Could you check a few things on this model? Use its own coordinates, in mm. A direction names the side the tool comes from. Coordinates: 2 decimals unless noted, no trailing zeros. Order: outer loops, then holes, each group sorted by start corner. A loop starts at its lowest first (then second) coordinate and runs counter-clockwise, first axis right, second up.
```python
from build123d import *

# Parameters (mm, degrees)
SKETCH1_W                     = 52
SKETCH1_H                     = 24
SKETCH1_R                     = 8.25
BOSS_EXTRUDE1_DEPTH           = 12
SKETCH2_R                     = 1
CUT_EXTRUDE1_DEPTH            = 32.048349393
SKETCH3_R                     = 1.75
CUT_EXTRUDE2_DEPTH            = 1
CUT_EXTRUDE3_DEPTH            = 5
FILLET3_R                     = 0.5
CHAMFER1_SIZE                 = 2.5
SKETCH5_W                     = 14
SKETCH5_H                     = 8
CUT_EXTRUDE4_DEPTH            = 5
FILLET4_R                     = 0.5
SKETCH6_W                     = 6.3
SKETCH6_H                     = 6.3
BOSS_EXTRUDE2_DEPTH           = 12
CSK_FOR_M3_SFHCS1_D           = 3
CSK_FOR_M3_SFHCS1_CSINK_D     = 6.3
CSK_FOR_M3_SFHCS1_CSINK_ANGLE = 90
CSK_FOR_M3_SFHCS2_D           = 3
CSK_FOR_M3_SFHCS2_DEPTH       = 109.998865618
CSK_FOR_M3_SFHCS2_CSINK_D     = 6.3
CSK_FOR_M3_SFHCS2_CSINK_ANGLE = 90


with BuildPart() as part:
    # Sketch1 → Boss-Extrude1 (new body)
    with BuildSketch(Plane(origin=(0, 0, 0), x_dir=(1, 0, 0), z_dir=(0, 1, 0))):
        Rectangle(SKETCH1_W, SKETCH1_H)
        with Locations(Location((12.75, 0, 0), (0, 0, 270))):
            Circle(SKETCH1_R, mode=Mode.SUBTRACT)
        with Locations(Location((-12.75, 0, 0), (0, 0, 270))):
            Circle(SKETCH1_R, mode=Mode.SUBTRACT)
    extrude(amount=BOSS_EXTRUDE1_DEPTH)

    # Sketch2 → Cut-Extrude1 (cut, through all)
    with BuildSketch(Plane(origin=(0, 12, 0), x_dir=(1, 0, 0), z_dir=(0, 1, 0))):
        with Locations(Location((-21.35, 8.85, 0), (0, 0, 270))):
            Circle(SKETCH2_R)
        with Locations(Location((21.35, 8.85, 0), (0, 0, 270))):
            Circle(SKETCH2_R)
        with Locations(Location((21.35, -8.85, 0), (0, 0, 270))):
            Circle(SKETCH2_R)
        with Locations(Location((-21.35, -8.85, 0), (0, 0, 270))):
            Circle(SKETCH2_R)
    extrude(amount=-CUT_EXTRUDE1_DEPTH, mode=Mode.SUBTRACT)

    # Sketch3 → Cut-Extrude2 (cut)
    with BuildSketch(Plane(origin=(0, 12, 0), x_dir=(1, 0, 0), z_dir=(0, 1, 0))):
        with Locations(Location((-21.35, 8.85, 0), (0, 0, 270))):
            Circle(SKETCH3_R)
        with Locations(Location((21.35, 8.85, 0), (0, 0, 270))):
            Circle(SKETCH3_R)
        with Locations(Location((21.35, -8.85, 0), (0, 0, 270))):
            Circle(SKETCH3_R)
        with Locations(Location((-21.35, -8.85, 0), (0, 0, 270))):
            Circle(SKETCH3_R)
    extrude(amount=-CUT_EXTRUDE2_DEPTH, mode=Mode.SUBTRACT)

    # Sketch4 → Cut-Extrude3 (cut)
    with BuildSketch(Plane.XZ):
        Polygon((-6, -5), (-6, -12), (6, -12), (6, -5), (0, -5), align=None)
    extrude(amount=-CUT_EXTRUDE3_DEPTH, mode=Mode.SUBTRACT)

    # Fillet3
    fillet3_edges = [part.edges().sort_by_distance(p)[0] for p in [
        (-6, 2.5, -5),
        (6, 5, -8.5),
        (6, 2.5, -5),
        (-6, 5, -8.5),
        (0, 5, -5),
    ]]
    fillet(fillet3_edges, radius=FILLET3_R)

    # Chamfer1
    chamfer1_edges = [part.edges().sort_by_distance(p)[0] for p in [
        (26, 6, 12),
        (-26, 6, 12),
        (-26, 6, -12),
        (26, 6, -12),
    ]]
    chamfer(chamfer1_edges, length=CHAMFER1_SIZE)

    # Sketch5 → Cut-Extrude4 (cut)
    with BuildSketch(Plane.XZ):
        with Locations((0, 12)):
            Rectangle(SKETCH5_W, SKETCH5_H)
    extrude(amount=-CUT_EXTRUDE4_DEPTH, mode=Mode.SUBTRACT)

    # Fillet4
    fillet4_edges = [part.edges().sort_by_distance(p)[0] for p in [
        (-7, 2.5, 8),
        (7, 5, 10),
        (0, 5, 8),
        (-7, 5, 10),
        (7, 2.5, 8),
    ]]
    fillet(fillet4_edges, radius=FILLET4_R)

    # Sketch6 → Boss-Extrude2 (add)
    with BuildSketch(Plane(origin=(0, 12, 0), x_dir=(1, 0, 0), z_dir=(0, 1, 0))):
        with Locations((-29.15, 0)):
            Rectangle(SKETCH6_W, SKETCH6_H)
        with Locations((29.15, 0)):
            Rectangle(SKETCH6_W, SKETCH6_H)
    extrude(amount=-BOSS_EXTRUDE2_DEPTH)

    # CSK for M3 SFHCS1 (through all)
    with Locations(Plane(origin=(1490.377712475, 12, 7.825775805), x_dir=(0.766044443118983, 0, -0.6427876096865334), z_dir=(0, 1, 0))):
        with Locations((-1114.335057549, 945.253960578), (-1158.995448583, 982.728478223)):
            CounterSinkHole(CSK_FOR_M3_SFHCS1_D / 2, CSK_FOR_M3_SFHCS1_CSINK_D / 2, counter_sink_angle=CSK_FOR_M3_SFHCS1_CSINK_ANGLE)

    # CSK for M3 SFHCS2
    with Locations(Plane(origin=(-1373.834887972, 567.783106147, 105.616816862), x_dir=(-0.6343091461006837, 0.5606811628058592, -0.5322485705454655), z_dir=(-0.42950668912891715, -0.8280317830099698, -0.3603989044362456))):
        with Locations((-1114.335057549, 945.253960578), (-1158.995448583, 982.728478223)):
            CounterSinkHole(CSK_FOR_M3_SFHCS2_D / 2, CSK_FOR_M3_SFHCS2_CSINK_D / 2, depth=CSK_FOR_M3_SFHCS2_DEPTH, counter_sink_angle=CSK_FOR_M3_SFHCS2_CSINK_ANGLE)


solid = part.part
```
Item 1: I need wall thicknesses on line 1 (X direction, y = 5.25, z = 8.85); line 2 (X direction, y = 8.75, z = 0); line 3 (X direction, y = 7.25, z = 3). Which ranges of each line are inside material? Lowest first, please.
Item 2: Thinking about a two-plate mould opening in X: for faces 1 (the face through (31.5, 12, -2.5)), 2 (the face through (-26, 6, -6)), 3 (the face through (-27.976, 0.505, 0.934)), which applies, +X half, -X half, draft (parallel to the pull), parting line (faces both ways), or undercut?
Item 3: Which directions (+Z, -Z, +X, -X, +Y, -Y) give clear straight access to the entire face, cutting with the end or side of a thin tool? Please do faces 4 (the face through (29, 6, -3.15)), 5 (the face through (-26, 6, 6)), 6 (the face through (-7, 2, 10)), 7 (the face through (19.8, 11.51, 9.66)), 8 (the face through (-29, 6, -3.15)).
Item 4: For pin 1 Ø7 at (y, z) = (6.5, 6) entering from -X; pin 2 Ø3 at (y, z) = (10, -5) entering from -X; pin 3 Ø5 at (x, y) = (29.5, 3.5) entering from +Z; pin 4 Ø4 at (x, z) = (-29.15, 0) entering from +Y, each with a flat end and sliding along its axis, tell me the tip position at first contact or that it passes through.
Item 5: Suppose I cut it at A-A (x = -12.75). List the corners of the cut face in (y, z) for me, and give its area (3 significant figures).
Item 6: Suppose I cut it at B-B (y = 9). Count the separate pieces of the cut face and the enclosed holes in it, and give its area (3 significant figures).
Geometry results:
1. line 1: x = -26 to -22.35, -20.35 to 20.35, 22.35 to 26
1. line 2: x = -32.3 to -30.65, -27.65 to -21, -4.5 to 4.5, 21 to 27.65, 30.65 to 32.3
1. line 3: x = -32.3 to -27.6, -24.39 to -20.44, -5.06 to 5.06, 20.44 to 32.3
2. face 1: draft
2. face 2: -X half
2. face 3: undercut
3. face 4: -Z, +X, +Y, -Y
3. face 5: +Z, -X, +Y, -Y
3. face 6: +Z, -Y
3. face 7: +Y
3. face 8: -Z, -X, +Y, -Y
4. pin 1: stops at x = -32.3
4. pin 2: stops at x = -26
4. pin 3: stops at z = 3.15
4. pin 4: stops at y = 10.85
5. outline: (0, -12) - (12, -12) - (12, -8.25) - (0, -8.25) - close; (0, 8.25) - (12, 8.25) - (12, 12) - (0, 12) - close
5. area: 90.0 mm2
6. separate pieces: 1
6. enclosed holes: 8
6. area: 853 mm2
